Source: three-view drawing plus pictorial views. Frame: mm from the lowest corner of the part. Coordinates: 2 decimals unless noted, no trailing zeros. Loops run counter-clockwise (first coordinate to the right, second up) from the corner with the lowest first, then second, coordinate; pieces in that order, holes last. Notation, with made-up numbers: (77.5, 38) - (84.5, 38) arc R21 cw to (84.5, 75) - close; hole circle Ø1 at (63.5, -4.5). An arc over 180 degrees is marked (long way). Answer as CSV lines item,"result". Start each with the question number.
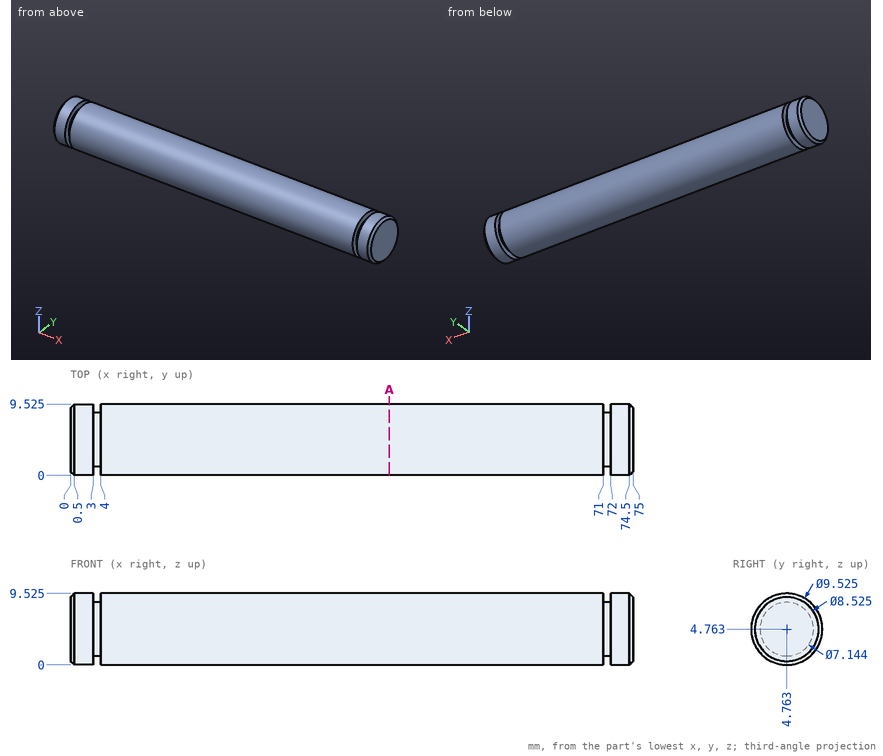
Item 1: Contact query for flat-ended pins moving along their axis: P1, Ø1.5, axis at x = 28.5, z = 2.5, coming from the -Y side; P2, Ø3, axis at x = 18.5, z = 7.5, coming from the +Y side; P3, Ø1, axis at x = 53.5, y = 3.5, coming from the -Z side. Output: stop coordinate, or through.
Item 2: Material intervals for probe 1 along X at (y, z) = (8.75, 6.25); probe 2 along Y at (x, z) = (56, 4.5); probe 3 along Z at (x, y) = (44, 8.5) (1 decimal), sorted ascending.
Item 3: Section query A-A, the plane x = 42.5. Output: boundary loops of the cut face in (y, z) (1 decimal).
Response values:
1,P1,"stops at y = 0.25"
1,P2,"stops at y = 9.36"
1,P3,"stops at z = 0.06"
2,probe 1,"x = 0 to 3, 4 to 71, 72 to 75"
2,probe 2,"y = 0.01 to 9.52"
2,probe 3,"z = 1.8 to 7.7"
3,outline,"circle Ø9.5 at (4.8, 4.8)"
